Verification items for the finished model (mm, model axes). Coordinates: 2 decimals unless noted, no trailing zeros. Write each loop counter-clockwise with the first axis right and the second up, starting at its lowest first coordinate (ties: lowest second). Pieces come first, ordered by that corner, then holes. Notation, with made-up numbers: (63, 10) -> (99, 10) arc R16 cw to (99, 37) -> close; hole circle Ø3 at (2, 11.25). An arc over 180 degrees is marked (long way). Answer in a Markdown table with one row per item.
```python
from build123d import *

# Parameters (mm, degrees)
SKETCH1_W           = 419
SKETCH1_H           = 303
BOSS_EXTRUDE1_DEPTH = 4
SKETCH2_W           = 119
SKETCH2_H           = 30
SKETCH2_W_2         = 109
CUT_EXTRUDE1_DEPTH  = 4
SKETCH3_R           = 2
CUT_EXTRUDE2_DEPTH  = 259.570106548
SKETCH4_R           = 2
CUT_EXTRUDE3_DEPTH  = 259.570106548


with BuildPart() as part:
    # Sketch1 → Boss-Extrude1 (new body)
    with BuildSketch(Plane.XY):
        Rectangle(SKETCH1_W, SKETCH1_H)
    extrude(amount=BOSS_EXTRUDE1_DEPTH)

    # Sketch2 → Cut-Extrude1 (cut)
    with BuildSketch(Plane(origin=(0, 0, 0), x_dir=(-1, 0, 0), z_dir=(0, 0, -1))):
        with Locations((-150, -136.5)):
            Rectangle(SKETCH2_W, SKETCH2_H)
        with Locations((155, -136.5)):
            Rectangle(SKETCH2_W_2, SKETCH2_H)
    extrude(amount=-CUT_EXTRUDE1_DEPTH, mode=Mode.SUBTRACT)

    # Sketch3 → Cut-Extrude2 (cut, through all)
    with BuildSketch(Plane(origin=(0, 0, 0), x_dir=(-1, 0, 0), z_dir=(0, 0, -1))):
        with Locations((-49.983602513, -136.5)):
            Circle(SKETCH3_R)
        with Locations((52.125756906, -136.5)):
            Circle(SKETCH3_R)
    extrude(amount=-CUT_EXTRUDE2_DEPTH, mode=Mode.SUBTRACT)

    # Sketch4 → Cut-Extrude3 (cut, through all)
    with BuildSketch(Plane(origin=(0, 0, 0), x_dir=(-1, 0, 0), z_dir=(0, 0, -1))):
        with Locations((199.5, -111.5)):
            Circle(SKETCH4_R)
        with Locations((199.5, -96.5)):
            Circle(SKETCH4_R)
    extrude(amount=-CUT_EXTRUDE3_DEPTH, mode=Mode.SUBTRACT)


solid = part.part
```
1. Thickness scan on line 1 (Y direction, x = -199.5, z = 1.1); line 2 (X direction, y = -136.5, z = 2); line 3 (Y direction, x = -166, z = 1.4). Record the ranges inside material, lowest first. Write a range as from..to.
Geometry says:
| item | result |
|---|---|
| line 1 | -121.5..-113.5, -109.5..-98.5, -94.5..151.5 |
| line 2 | -100.5..-54.13, -50.13..47.98, 51.98..90.5 |
| line 3 | -121.5..151.5 |
2. Section check A-A, the plane z = 2.6. Record the boundary of the cut face in (x, y).
Geometry says:
| item | result |
|---|---|
| outline | (-209.5, -121.5) -> (-100.5, -121.5) -> (-100.5, -151.5) -> (90.5, -151.5) -> (90.5, -121.5) -> (209.5, -121.5) -> (209.5, 151.5) -> (-209.5, 151.5) -> close; hole circle Ø4 at (-199.5, -111.5); hole circle Ø4 at (-199.5, -96.5); hole circle Ø4 at (-52.13, -136.5); hole circle Ø4 at (49.98, -136.5) |
3. Section check B-B, the plane x = -113. Record the boundary of the cut face in (y, z), plus the area to 3 significant figures.
Geometry says:
| item | result |
|---|---|
| outline | (-121.5, 0) -> (151.5, 0) -> (151.5, 4) -> (-121.5, 4) -> close |
| area | 1,090 mm^2 |
4. Depth check by flat-ended pin: P1, Ø2, axis at y = -132.5, z = 2.5, coming from the -X side; P2, Ø6, axis at x = -122, y = 120, coming from the -Z side; P3, Ø1.2, axis at x = 157.5, z = 2.5, coming from the -Y side; P4, Ø1.2, axis at y = -139, z = 2.5, coming from the +X side. Enter the tip coordinate at first touch or a pass-through.
Geometry says:
| item | result |
|---|---|
| P1 | x = -100.5 |
| P2 | z = 0 |
| P3 | y = -121.5 |
| P4 | x = 90.5 |
